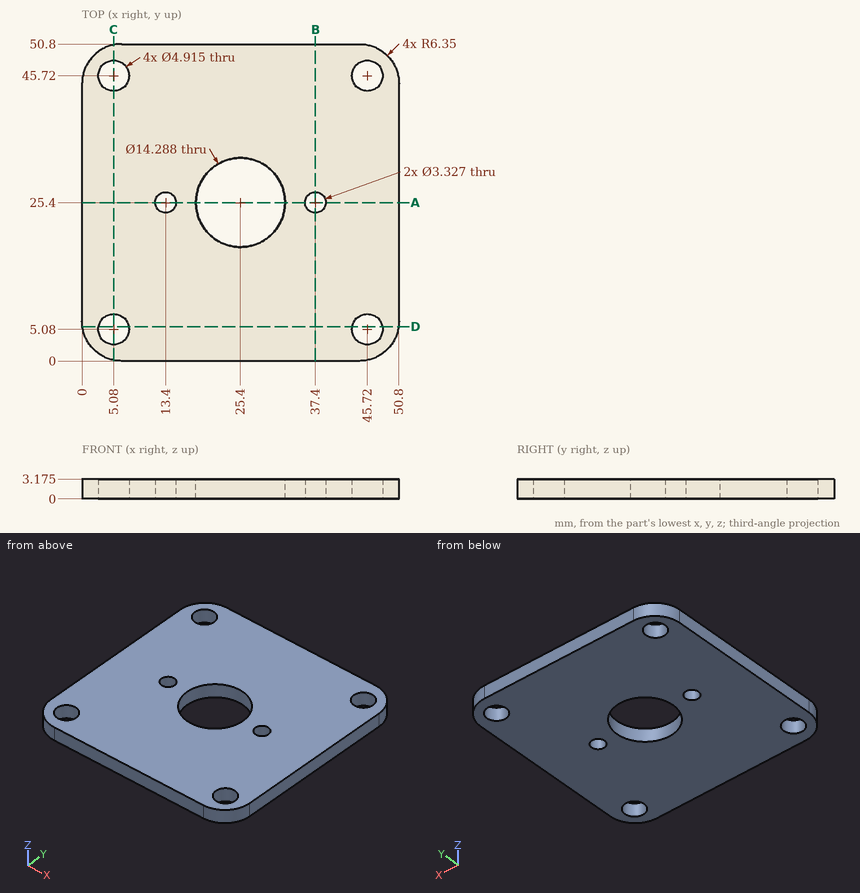
Part print with two shaded views. Sizes in mm from the minimum x, y, z corner. Round coordinates to 2 decimals unless told otherwise and drop trailing zeros. Order: outer loops, then holes, each group sorted by start corner. A loop starts at its lowest first (then second) coordinate and runs counter-clockwise, first axis right, second up. Notation, with made-up numbers: (45.25, 60) - (62.25, 60) arc R16 cw to (62.25, 67) - close; hole circle Ø3 at (3, -21.5). An arc over 180 degrees is marked (long way). Answer as CSV lines item,"result". Start each with the question number.
1. Saw through at C-C, the plane x = 5.08. Write the cut outline in (y, z) (1 decimal).
2. Saw through at A-A, the plane y = 25.4. Write the cut outline in (x, z) (1 decimal).
3. Drill centre lines: L1, parallel to X at y = 25.4, z = 1.1; L2, parallel to Y at x = 6.5, z = 1.5 (1 decimal); L3, parallel to Y at x = 5.08, z = 1.6. Where is each one in solid material? Low to high. Write a range as [from, to].
4. Saw through at D-D, the plane y = 5.5. Write the cut outline in (x, z) (1 decimal).
5. Saw through at B-B, the plane x = 37.4. Write the cut outline in (y, z) (1 decimal).
Model answer:
1,outline,"(0.1, 0) - (2.6, 0) - (2.6, 3.2) - (0.1, 3.2) - close; (7.5, 0) - (43.3, 0) - (43.3, 3.2) - (7.5, 3.2) - close; (48.2, 0) - (50.7, 0) - (50.7, 3.2) - (48.2, 3.2) - close"
2,outline,"(0, 0) - (11.7, 0) - (11.7, 3.2) - (0, 3.2) - close; (15.1, 0) - (18.3, 0) - (18.3, 3.2) - (15.1, 3.2) - close; (32.5, 0) - (35.7, 0) - (35.7, 3.2) - (32.5, 3.2) - close; (39.1, 0) - (50.8, 0) - (50.8, 3.2) - (39.1, 3.2) - close"
3,L1,"x = [0, 11.74], [15.06, 18.26], [32.54, 35.74], [39.06, 50.8]"
3,L2,"y = [0, 3.1], [7.1, 43.7], [47.7, 50.8]"
3,L3,"y = [0.13, 2.62], [7.54, 43.26], [48.18, 50.67]"
4,outline,"(0.1, 0) - (2.7, 0) - (2.7, 3.2) - (0.1, 3.2) - close; (7.5, 0) - (43.3, 0) - (43.3, 3.2) - (7.5, 3.2) - close; (48.1, 0) - (50.7, 0) - (50.7, 3.2) - (48.1, 3.2) - close"
5,outline,"(0, 0) - (23.7, 0) - (23.7, 3.2) - (0, 3.2) - close; (27.1, 0) - (50.8, 0) - (50.8, 3.2) - (27.1, 3.2) - close"
